Here's how the part is built. I have some questions about the finished solid (model axes, mm). A direction names the side the tool comes from. Round coordinates to 2 decimals unless told otherwise and drop trailing zeros. Loops run counter-clockwise (first coordinate to the right, second up) from the corner with the lowest first, then second, coordinate; pieces in that order, holes last. Notation, with made-up numbers: M 83,-8 L 97,-8 A15 ccw 97,21 Z; hole C 53,13.25 d7. An arc over 180 degrees is marked long. Answer as a JSON object with one key per item and string values.
from build123d import *

# Parameters (mm, degrees)
BOSS_EXTRUDE1_DEPTH = 152.4
SKETCH2_R           = 9.525
SKETCH2_R_2         = 6.096
SKETCH2_R_3         = 7.62
CUT_EXTRUDE1_DEPTH  = 152.4
SKETCH3_R           = 3.175
BOSS_EXTRUDE2_DEPTH = 12.7
SKETCH4_R           = 3.175
BOSS_EXTRUDE3_DEPTH = 12.7
BOSS_EXTRUDE5_DEPTH = 12.7
BOSS_EXTRUDE6_DEPTH = 12.7


with BuildPart() as part:
    # Sketch1 → Boss-Extrude1 (new body)
    with BuildSketch(Plane.XY):
        Polygon((0, 0), (38.1, 0), (152.4, -63.5), (152.4, -57.15), (38.1, 6.35), (0, 6.35), align=None)
    extrude(amount=BOSS_EXTRUDE1_DEPTH)

    # Sketch2 → Cut-Extrude1 (cut)
    with BuildSketch(Plane(origin=(11.681603774, 21.026886792, 0), x_dir=(0.874157276, -0.485642931, 0), z_dir=(0.485642931, 0.874157276, 0))):
        with Locations((87.371559607, -120.65)):
            Circle(SKETCH2_R)
        with Locations((87.371559607, -76.2)):
            Circle(SKETCH2_R_2)
        with Locations((87.371559607, -31.75)):
            Circle(SKETCH2_R_3)
    extrude(amount=-CUT_EXTRUDE1_DEPTH, mode=Mode.SUBTRACT)

    # Sketch3 → Boss-Extrude2 (add)
    with BuildSketch(Plane.XZ):
        with Locations((12.7, 6.35)):
            Circle(SKETCH3_R)
        with Locations((12.7, 146.05)):
            Circle(SKETCH3_R)
    extrude(amount=BOSS_EXTRUDE2_DEPTH)

    # Sketch4 → Boss-Extrude3 (add)
    with BuildSketch(Plane(origin=(8.985849057, 16.174528302, 0), x_dir=(0.874157276, -0.485642931, 0), z_dir=(-0.485642931, -0.874157276, 0))):
        with Locations((151.359895011, 6.35)):
            Circle(SKETCH4_R)
        with Locations((151.359895011, 146.05)):
            Circle(SKETCH4_R)
    extrude(amount=BOSS_EXTRUDE3_DEPTH)

    # Sketch7 → Boss-Extrude5 (add)
    with BuildSketch(Plane.XY.offset(152.4)):
        Polygon((0, 0), (0, 6.35), (38.1, 6.35), (152.4, -57.15), (152.4, -63.5), (38.1, 0), align=None)
    extrude(amount=BOSS_EXTRUDE5_DEPTH)

    # Sketch8 → Boss-Extrude6 (add)
    with BuildSketch(Plane(origin=(0, 0, 0), x_dir=(-1, 0, 0), z_dir=(0, 0, -1))):
        Polygon((0, 0), (-38.1, 0), (-152.4, -63.5), (-152.4, -57.15), (-38.1, 6.35), (0, 6.35), align=None)
    extrude(amount=BOSS_EXTRUDE6_DEPTH)


solid = part.part
Item 1: I want a section at B-B, the plane x = 12.7. Please give me the cut outline in (y, z) (3 decimals), then the cut area to 3 significant figures.
Resolved:
{"outline": "M -12.7,3.175 L 0,3.175 L 0,-12.7 L 6.35,-12.7 L 6.35,165.1 L 0,165.1 L 0,149.225 L -12.7,149.225 L -12.7,142.875 L 0,142.875 L 0,9.525 L -12.7,9.525 Z", "area": "1,290 mm²"}
Item 2: I want a section at D-D, the plane z = 74. Please give me the cut outline in (x, y).
Resolved:
{"outline": "M 0,0 L 38.1,0 L 80.39,-23.5 L 83.09,-18.64 L 38.1,6.35 L 0,6.35 Z; M 90.33,-29.02 L 152.4,-63.5 L 152.4,-57.15 L 93.03,-24.17 Z"}
Item 3: I want a section at C-C, the plane z = 6.35. Please give me the cut outline in (x, y) (3 decimals).
Resolved:
{"outline": "M 0,0 L 9.525,0 L 9.525,-12.7 L 15.875,-12.7 L 15.875,0 L 38.1,0 L 138.523,-55.79 L 132.355,-66.892 L 137.906,-69.976 L 144.074,-58.874 L 152.4,-63.5 L 152.4,-57.15 L 38.1,6.35 L 0,6.35 Z"}
Item 4: If we mould it in two halves opening along Z, with no side actions, what happens to faces 4 (the face through (10.36, -6.261, 8.496)), 5 (the face through (71, -18, 165.1)), 6 (the face through (19, 6.35, 77))? For each: pulls with the +Z half, pulls with the -Z half, needs draft (parallel to the pull), parting line crosses it, or undercut.
Resolved:
{"face 4": "undercut", "face 5": "pulls with the +Z half", "face 6": "needs draft"}
Item 5: I want a section at A-A, the plane z = 123.5. Please give me the cut outline in (x, y), then the cut area to 3 significant figures.
Resolved:
{"outline": "M 0,0 L 38.1,0 L 77.42,-21.84 L 80.11,-16.99 L 38.1,6.35 L 0,6.35 Z; M 93.31,-30.67 L 152.4,-63.5 L 152.4,-57.15 L 96,-25.82 Z", "area": "867 mm²"}
Item 6: On a 3-axis mill with a long thin cutter (end or side, diameter ignored), from which of +Z, -Z, +X, -X, +Y, -Y can I reach the whole of each face in a straight line? I mean faces 1 (the face through (0, 3, 77)), 2 (the face through (12.3, -6.3, 149.2)), 3 (the face through (13, -12.7, 6)). Say none if no direction works.
Resolved:
{"face 1": "+Z, -Z, -X, +Y, -Y", "face 2": "-Y", "face 3": "+Z, -Z, -X, -Y"}
Item 7: I'm going to push flat-ended pins straight in: pin 1 Ø3 at (y, z) = (-45, 98.5) entering from +X; pin 2 Ø7 at (x, z) = (13.5, 7.5) entering from -Y; pin 3 Ø2 at (y, z) = (-22, 141.5) entering from -X. Where does each tip first touch, or does it pass through?
Resolved:
{"pin 1": "x = 133.23", "pin 2": "y = -12.7", "pin 3": "x = 75.9"}
Item 8: Please list where these lines run through material, in increasing order: probe 1 along Y at (x, z) = (24, 49); probe 2 along Y at (x, z) = (79.5, 2.5); probe 3 along X at (y, z) = (-21.5, 2). Write a range as from..to.
Resolved:
{"probe 1": "0..6.35", "probe 2": "-23..-16.65", "probe 3": "76.8..88.23"}
